```python
from build123d import *

# Parameters (mm, degrees)
F0_W     = 49.110298
F0_H     = 61.184842
F1_DEPTH = 50.8
F2_W     = 11
F2_H     = 11
F3_DEPTH = 45.72
F6_DEPTH = 50.8
F7_DEPTH = 50.8


with BuildPart() as f1:
    # F0 (on Top) → F1 (new body)
    with BuildSketch(Plane.XY):
        Rectangle(F0_W, F0_H)
    extrude(amount=F1_DEPTH)

    # F2 (on face) → F3 (cut)
    with BuildSketch(Plane.XY.offset(50.8)):
        Rectangle(F2_W, F2_H)
    extrude(amount=-F3_DEPTH, mode=Mode.SUBTRACT)

    # F4 (on Front) → F6 (cut)
    with BuildSketch(Plane.XZ):
        Polygon((-2.50393, 23.495), (-2.50393, 14.605), (0, 14.605), (2.50393, 14.605), (2.50393, 23.495), align=None)
    extrude(amount=-F6_DEPTH, mode=Mode.SUBTRACT)

    # F5 (on face) → F7 (cut)
    with BuildSketch(Plane.XZ.offset(30.592421)):
        with BuildLine():
            ThreePointArc((4.445, 17.878173), (-3.14309, 21.021263), (0, 13.433173))
            ThreePointArc((0, 13.433173), (3.14309, 14.735084), (4.445, 17.878173))
        make_face()
    extrude(amount=-F7_DEPTH, mode=Mode.SUBTRACT)


solid = f1.part
```
Geometry check sheet. Reference: the model listing, model coordinates, mm. A direction names the side the tool comes from. Coordinates: 2 decimals unless noted, no trailing zeros. Order: outer loops, then holes, each group sorted by start corner. A loop starts at its lowest first (then second) coordinate and runs counter-clockwise, first axis right, second up.
Item 1: Scan lines: line 1 along Y through (x, z) = (2.5, 27.5); line 2 along Z through (x, y) = (0, -25.5); line 3 along X through (y, z) = (25, 19.5). Record each from-to range of solid material in increasing order.
Item 2: Tool access check on faces 4 (the flat face through (3, 20.208, 17)), 5 (the flat face through (0, 25, 14.605)), 6 (the flat face through (-24.555, 0, 25)), 7 (the flat face through (0, 5.5, 28)), 8 (the flat face through (2.504, 23, 20)). Record the directions out of +Z, -Z, +X, -X, +Y, -Y that give a thin tool (end or side, any length) a straight path to the whole face; none if there is none.
Item 3: Mould release check, pull along Z, two halves, no side actions. Record for faces 1 (the flat face through (0, 0, 0)), 2 (the flat face through (24.555, 0, 25)), 3 (the flat face through (0, 18, 23.495)): released by +Z, released by -Z, zero draft, split by the parting line, or undercut.
Item 4: Section check A-A (z = 6). Enter the section's corners in (x, y).
Item 5: Section check C-C (z = 19). Enter the section's corners in (x, y), plus the area to 3 significant figures.
Item 6: Section check D-D (y = -19.5). Enter the section's corners in (x, z) (3 decimals), plus the area to 3 significant figures.
Item 7: Depth check by flat-ended pin: pin 1 (4 mm diameter, centred on x = -1.5, z = 19.5, fed in from -Y); pin 2 (5.5 mm diameter, centred on x = 2, y = -1.5, fed in from +Z). Enter the tip coordinate at first touch or a pass-through.
Item 8: Section check B-B (y = 12). Enter the section's corners in (x, z) (3 decimals).
Check sheet entries:
1. line 1: y = -30.59 to -5.5, 5.5 to 30.59
1. line 2: z = 0 to 13.43, 22.32 to 50.8
1. line 3: x = -24.56 to -2.5, 2.5 to 24.56
2. face 4: -Y
2. face 5: +Y, -Y
2. face 6: +Z, -Z, -X, +Y, -Y
2. face 7: +Z
2. face 8: +Y
3. face 1: released by -Z
3. face 2: zero draft
3. face 3: undercut
4. outline: (-24.56, -30.59) - (24.56, -30.59) - (24.56, 30.59) - (-24.56, 30.59) - close; hole (-5.5, -5.5) - (5.5, -5.5) - (5.5, 5.5) - (-5.5, 5.5) - close
5. outline: (-24.56, -30.59) - (-4.3, -30.59) - (-4.3, -5.5) - (-5.5, -5.5) - (-5.5, 5.5) - (-4.3, 5.5) - (-4.3, 20.21) - (-2.5, 20.21) - (-2.5, 30.59) - (-24.56, 30.59) - close; (2.5, 20.21) - (4.3, 20.21) - (4.3, 5.5) - (5.5, 5.5) - (5.5, -5.5) - (4.3, -5.5) - (4.3, -30.59) - (24.56, -30.59) - (24.56, 30.59) - (2.5, 30.59) - close
5. area: 2,490 mm2
6. outline: (-24.555, 0) - (24.555, 0) - (24.555, 50.8) - (-24.555, 50.8) - close; hole circle Ø8.89 at (0, 17.878)
6. area: 2,430 mm2
7. pin 1: stops at y = 20.21
7. pin 2: stops at z = 5.08
8. outline: (-24.555, 0) - (24.555, 0) - (24.555, 50.8) - (-24.555, 50.8) - close; hole (-2.504, 21.551) arc R4.445 ccw (long way) to (2.504, 21.551) - (2.504, 23.495) - (-2.504, 23.495) - close
